```python
from build123d import *

# Parameters (mm, degrees)
F0_R     = 76.2
F0_R_2   = 3.175
F1_DEPTH = 38.1


with BuildPart() as f1:
    # F0 (on Top) → F1 (new body)
    with BuildSketch(Plane.XY):
        Circle(F0_R)
        with Locations((-44.901281, -42.811689)):
            Circle(F0_R_2, mode=Mode.SUBTRACT)
        with Locations((0, -61.410408)):
            Circle(F0_R_2, mode=Mode.SUBTRACT)
        with Locations((44.901281, -42.811689)):
            Circle(F0_R_2, mode=Mode.SUBTRACT)
        with Locations((-63.5, 2.089592)):
            Circle(F0_R_2, mode=Mode.SUBTRACT)
        with Locations((-44.901281, 46.990872)):
            Circle(F0_R_2, mode=Mode.SUBTRACT)
        with Locations((63.5, 2.089592)):
            Circle(F0_R_2, mode=Mode.SUBTRACT)
        with Locations((0, 65.589592)):
            Circle(F0_R_2, mode=Mode.SUBTRACT)
        with Locations((44.901281, 46.990872)):
            Circle(F0_R_2, mode=Mode.SUBTRACT)
    extrude(amount=F1_DEPTH)


solid = f1.part
```
Could you check a few things on this model? Use its own coordinates, in mm. Give positions to 0.01 mm unless a question says otherwise; leave off trailing zeros. Order: outer loops, then holes, each group sorted by start corner. A loop starts at its lowest first (then second) coordinate and runs counter-clockwise, first axis right, second up.
Q1. If I drill on line 1 along X through (y, z) = (-41, 32); line 2 along Y through (x, z) = (65, 24); line 3 along Y through (x, z) = (-63, 3), over which ranges is the centre line in solid material (lowest first)?
Q2. We'd pull the mould along Y, two halves only. Please class faces 1 (the cylindrical face through (44.21, 43.89, 18.78)), 2 (the cylindrical face through (-60.47, 3.04, 18.78)), 3 (the flat face through (-1, 1, 38.1)), 4 (the cylindrical face through (-60.47, -46.367, 18.783)): +Y half, -Y half, draft (parallel to the pull), parting line (faces both ways), or undercut.
Q3. Suppose I cut it at B-B, the plane z = 14. Count the separate pieces of the cut face and the enclosed holes in it, and give its area (3 significant figures).
Q4. Suppose I cut it at D-D, the plane x = -46. Write out the boundary of the cut face in (y, z).
Q5. Suppose I cut it at A-A, the plane x = 0. Write out the boundary of the cut face in (y, z), and give its area (3 significant figures).
Q6. Suppose I cut it at C-C, the plane x = 63.5. Write out the boundary of the cut face in (y, z).
Q7. I'm going to push flat-ended pins straight in: P1, Ø10, axis at y = -34, z = 28, coming from the +X side; P2, Ø5.5, axis at x = 63.5, y = 2.09, coming from the -Z side; P3, Ø3, axis at x = -19.5, z = 27, coming from the +Y side; P4, Ø5, axis at x = 58.5, z = 13.5, coming from the -Y side. Where does each tip first touch, or does it pass through?
Solution:
1. line 1: x = -64.23 to -47.51, -42.29 to 42.29, 47.51 to 64.23
1. line 2: y = -39.77 to -0.71, 4.89 to 39.77
1. line 3: y = -42.87 to -1.05, 5.22 to 42.87
2. face 1: undercut
2. face 2: undercut
2. face 3: draft
2. face 4: parting line
3. separate pieces: 1
3. enclosed holes: 8
3. area: 18,000 mm2
4. outline: (-60.75, 0) - (-45.79, 0) - (-45.79, 38.1) - (-60.75, 38.1) - close; (-39.83, 0) - (44.01, 0) - (44.01, 38.1) - (-39.83, 38.1) - close; (49.97, 0) - (60.75, 0) - (60.75, 38.1) - (49.97, 38.1) - close
5. outline: (-76.2, 0) - (-64.59, 0) - (-64.59, 38.1) - (-76.2, 38.1) - close; (-58.24, 0) - (62.41, 0) - (62.41, 38.1) - (-58.24, 38.1) - close; (68.76, 0) - (76.2, 0) - (76.2, 38.1) - (68.76, 38.1) - close
5. area: 5,320 mm2
6. outline: (-42.12, 0) - (-1.09, 0) - (-1.09, 38.1) - (-42.12, 38.1) - close; (5.26, 0) - (42.12, 0) - (42.12, 38.1) - (5.26, 38.1) - close
7. P1: stops at x = 70.47
7. P2: passes through
7. P3: stops at y = 74.04
7. P4: stops at y = -51.68
